Input: part model. Units: mm. Frame: model coordinates. Coordinates: 2 decimals unless noted, no trailing zeros. Write each loop counter-clockwise with the first axis right and the second up, starting at its lowest first coordinate (ties: lowest second). Pieces come first, ordered by that corner, then holes.
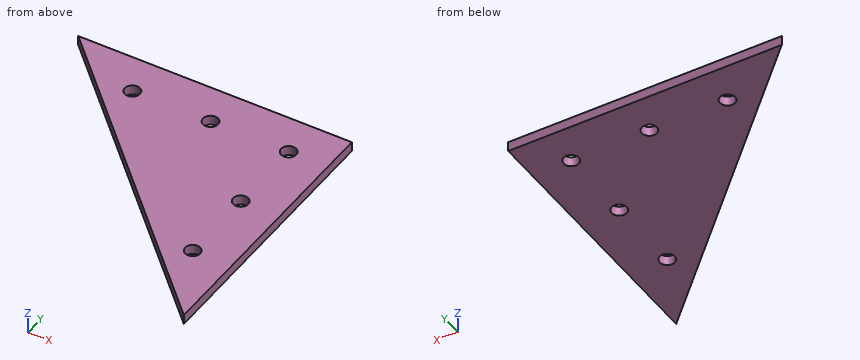
from build123d import *

# Parameters (mm, degrees)
SKETCH1_R           = 2.4765
BOSS_EXTRUDE1_DEPTH = 1.5875


with BuildPart() as part:
    # Sketch1 → Boss-Extrude1 (new body, symmetric)
    with BuildSketch(Plane.XY):
        Polygon((-44.45, 44.45), (44.45, 44.45), (44.45, -44.45), align=None)
        with Locations((6.35, 31.75)):
            Circle(SKETCH1_R, mode=Mode.SUBTRACT)
        with Locations((31.75, 31.75)):
            Circle(SKETCH1_R, mode=Mode.SUBTRACT)
        with Locations((31.75, 6.35)):
            Circle(SKETCH1_R, mode=Mode.SUBTRACT)
        with Locations((31.75, -19.05)):
            Circle(SKETCH1_R, mode=Mode.SUBTRACT)
        with Locations((-19.05, 31.75)):
            Circle(SKETCH1_R, mode=Mode.SUBTRACT)
    extrude(amount=BOSS_EXTRUDE1_DEPTH, both=True)


solid = part.part
Item 1: Section query C-C, the plane z = 0.7. Return loops of the section in (x, y), then the cut area to 3 significant figures.
Item 2: Pin query (flat end, axial travel): pin 1 Ø3 at (x, y) = (31.75, 6.35) entering from -Z; pin 2 Ø8 at (x, y) = (6.35, 31.75) entering from +Z; pin 3 Ø1 at (x, z) = (-7, 0.5) entering from -Y. Return the tip coordinate at first contact, or that it passes through.
Item 3: Section query D-D, the plane x = 31.75. Return loops of the section in (y, z).
Item 4: Section query B-B, the plane x = -19.05. Return loops of the section in (y, z), then the cut area to 3 significant figures.
Item 5: Material intervals for line 1 (Y direction, x = 31.75, z = -0.25); line 2 (X direction, y = 34, z = 0); line 3 (X direction, y = 32, z = 1.15), sorted ascending.
Item 6: Section query A-A, the plane y = 6.35. Return loops of the section in (x, z).
The answers:
1. outline: (-44.45, 44.45) - (44.45, -44.45) - (44.45, 44.45) - close; hole circle Ø4.95 at (-19.05, 31.75); hole circle Ø4.95 at (6.35, 31.75); hole circle Ø4.95 at (31.75, -19.05); hole circle Ø4.95 at (31.75, 6.35); hole circle Ø4.95 at (31.75, 31.75)
1. area: 3,860 mm2
2. pin 1: passes through
2. pin 2: stops at z = 1.59
2. pin 3: stops at y = 6.5
3. outline: (-31.75, -1.59) - (-21.53, -1.59) - (-21.53, 1.59) - (-31.75, 1.59) - close; (-16.57, -1.59) - (3.87, -1.59) - (3.87, 1.59) - (-16.57, 1.59) - close; (8.83, -1.59) - (29.27, -1.59) - (29.27, 1.59) - (8.83, 1.59) - close; (34.23, -1.59) - (44.45, -1.59) - (44.45, 1.59) - (34.23, 1.59) - close
4. outline: (19.05, -1.59) - (29.27, -1.59) - (29.27, 1.59) - (19.05, 1.59) - close; (34.23, -1.59) - (44.45, -1.59) - (44.45, 1.59) - (34.23, 1.59) - close
4. area: 64.9 mm2
5. line 1: y = -31.75 to -21.53, -16.57 to 3.87, 8.83 to 29.27, 34.23 to 44.45
5. line 2: x = -34 to -20.08, -18.02 to 5.32, 7.38 to 30.72, 32.78 to 44.45
5. line 3: x = -32 to -21.51, -16.59 to 3.89, 8.81 to 29.29, 34.21 to 44.45
6. outline: (-6.35, -1.59) - (29.27, -1.59) - (29.27, 1.59) - (-6.35, 1.59) - close; (34.23, -1.59) - (44.45, -1.59) - (44.45, 1.59) - (34.23, 1.59) - close
